Design review of the part built by this model. Coordinates are the model's own, in mm. Give positions to 0.01 mm unless a question says otherwise; leave off trailing zeros. Order: outer loops, then holes, each group sorted by start corner. A loop starts at its lowest first (then second) coordinate and runs counter-clockwise, first axis right, second up. Notation, with made-up numbers: M 5,72 L 9,72 A20 cw 9,76 Z; hole C -14.5,-39.5 d10. An arc over 180 degrees is marked long. Answer as a JSON object with one key per item and string values.
from build123d import *

# Parameters (mm, degrees)
F1_DEPTH = 40
F3_DEPTH = 494


with BuildPart() as f1:
    # F0 (on Front) → F1 (new body)
    with BuildSketch(Plane.XZ):
        with BuildLine():
            add(Edge.make_bspline(
                [(0, 252), (15.8393937026, 187.6250477101), (73.9196968513, 93.8125238551), (132, 0)],
                knots=[0.3599862205, 0.3599862205, 0.3599862205, 0.3599862205, 1, 1, 1, 1], degree=3))
            Line((132, 0), (158, 0))
            add(Edge.make_bspline(
                [(290, 252), (274.1606062974, 187.6250477101), (216.0803031487, 93.8125238551), (158, 0)],
                knots=[0.3599862205, 0.3599862205, 0.3599862205, 0.3599862205, 1, 1, 1, 1], degree=3))
            Line((290, 252), (290, 342))
            Line((290, 342), (272, 360))
            Line((272, 360), (18, 360))
            Line((18, 360), (0, 342))
            Line((0, 342), (0, 252))
        make_face()
    extrude(amount=F1_DEPTH)

    # F2 (on face) → F3 (cut)
    with BuildSketch(Plane.XY.offset(360)):
        Polygon((-17.8489275277, 46.4588217437), (-17.8489275277, -40), (145, 0), (310.4465901852, -40), (307.7366054058, 46.4588217437), align=None)
    extrude(amount=-F3_DEPTH, mode=Mode.SUBTRACT)


solid = f1.part
(1) To check wall thickness, follow L1, parallel to Y at x = 210, z = 113.5; L2, parallel to X at y = -32, z = 24.5; L3, parallel to Y at x = 120.5, z = 108. State the ranges of each line that lie inside material, in increasing order. Write a range as from..to.
Checked values:
{"L1": "y = -40..-15.72", "L2": "x = 116.85..173.15", "L3": "y = -40..-6.02"}
(2) Insertion check: pin 1 (4 mm diameter, centred on x = 137, z = 163.5, fed in from +Y); pin 2 (3 mm diameter, centred on x = 117.5, y = -18.5, fed in from -Z); pin 3 (1 mm diameter, centred on x = 222, y = -26.5, fed in from -Z). Each pin has a flat end and moves straight along its axis. Give the tip position at first contact, or say it passes through.
Checked values:
{"pin 1": "stops at y = -1.47", "pin 2": "stops at z = 21.01", "pin 3": "stops at z = 104.65"}
(3) We need section A-A (z = 314.5). Write out the cut boundary in (x, y), plus the area to 3 significant figures.
Checked values:
{"outline": "M 0,-40 L 290,-40 L 290,-35.06 L 145,0 L 0,-35.62 Z", "area": "6,480 mm^2"}
